Could you check a few things on this model? Use its own coordinates, in mm. A direction names the side the tool comes from. Give positions to 0.01 mm unless a question says otherwise; leave off trailing zeros. Write each loop counter-clockwise with the first axis right and the second up, starting at its lowest first coordinate (ties: lowest second). Pieces come first, ordered by that corner, then holes. Notation, with made-up numbers: (43.5, -12.5) - (73.5, -12.5) arc R11 cw to (73.5, -7.5) - close; hole circle Ø8 at (79.25, 80). An arc over 180 degrees is marked (long way). Use one line per item in the form item = value.
```python
from build123d import *

# Parameters (mm, degrees)
SKETCH1_W           = 76
SKETCH1_H           = 50
BOSS_EXTRUDE1_DEPTH = 20
SKETCH2_W           = 47
SKETCH2_H           = 17
CUT_EXTRUDE1_DEPTH  = 76
SKETCH3_R           = 6.5
CUT_EXTRUDE2_DEPTH  = 2
SKETCH4_R           = 5
CUT_EXTRUDE3_DEPTH  = 2
SKETCH5_R           = 1.2
CUT_EXTRUDE4_DEPTH  = 2


with BuildPart() as part:
    # Sketch1 → Boss-Extrude1 (new body)
    with BuildSketch(Plane(origin=(0, 0, 0), x_dir=(1, 0, 0), z_dir=(0, 1, 0))):
        with Locations((11.529653553, 8.750876438)):
            Rectangle(SKETCH1_W, SKETCH1_H)
    extrude(amount=BOSS_EXTRUDE1_DEPTH)

    # Sketch2 → Cut-Extrude1 (cut)
    with BuildSketch(Plane.ZY.offset(26.470346447)):
        with Locations((-8.750876438, 10)):
            Rectangle(SKETCH2_W, SKETCH2_H)
    extrude(amount=-CUT_EXTRUDE1_DEPTH, mode=Mode.SUBTRACT)

    # Sketch3 → Cut-Extrude2 (cut)
    with BuildSketch(Plane(origin=(0, 0, -33.750876438), x_dir=(-1, 0, 0), z_dir=(0, 0, -1))):
        with Locations((10.970346447, 10)):
            Circle(SKETCH3_R)
        with Locations((-4.029653553, 10)):
            Circle(SKETCH3_R)
        with Locations((-19.029653553, 10)):
            Circle(SKETCH3_R)
        with Locations((-34.029653553, 10)):
            Circle(SKETCH3_R)
    extrude(amount=-CUT_EXTRUDE2_DEPTH, mode=Mode.SUBTRACT)

    # Sketch4 → Cut-Extrude3 (cut)
    with BuildSketch(Plane.XY.offset(16.249123562)):
        with Locations((-10.970346447, 10)):
            Circle(SKETCH4_R)
        with Locations((4.029653553, 10)):
            Circle(SKETCH4_R)
        with Locations((19.029653553, 10)):
            Circle(SKETCH4_R)
        with Locations((34.029653553, 10)):
            Circle(SKETCH4_R)
    extrude(amount=-CUT_EXTRUDE3_DEPTH, mode=Mode.SUBTRACT)

    # Sketch5 → Cut-Extrude4 (cut)
    with BuildSketch(Plane(origin=(0, 0, 0), x_dir=(-1, 0, 0), z_dir=(0, -1, 0))):
        with Locations(Location((-34.029653553, 20.750876438, 0), (0, 0, 90))):  # turned: the seam where the file's is
            Circle(SKETCH5_R)
        with Locations(Location((-19.029653553, 20.750876438, 0), (0, 0, 90))):  # turned: the seam where the file's is
            Circle(SKETCH5_R)
        with Locations(Location((-4.029653553, 20.750876438, 0), (0, 0, 90))):  # turned: the seam where the file's is
            Circle(SKETCH5_R)
        with Locations(Location((10.970346447, 20.750876438, 0), (0, 0, 90))):  # turned: the seam where the file's is
            Circle(SKETCH5_R)
        with Locations(Location((-19.029653553, 5.750876438, 0), (0, 0, 90))):  # turned: the seam where the file's is
            Circle(SKETCH5_R)
        with Locations(Location((-4.029653553, 5.750876438, 0), (0, 0, 90))):  # turned: the seam where the file's is
            Circle(SKETCH5_R)
        with Locations(Location((10.970346447, 5.750876438, 0), (0, 0, 90))):  # turned: the seam where the file's is
            Circle(SKETCH5_R)
        with Locations(Location((-34.029653553, 5.750876438, 0), (0, 0, 90))):  # turned: the seam where the file's is
            Circle(SKETCH5_R)
    extrude(amount=-CUT_EXTRUDE4_DEPTH, mode=Mode.SUBTRACT)


solid = part.part
```
1. If I drill on line 1 (Y direction, x = 21.5, z = 7); line 2 (Z direction, x = 30.5, y = 17.25); line 3 (Z direction, x = -1, y = 9.75), over which ranges is the centre line in solid material (lowest first)? Write a range as from..to.
Response values:
line_1 = 0..1.5, 18.5..20
line_2 = -33.75..-32.25, 14.75..16.25
line_3 = 14.75..16.25
2. If we mould it in two halves opening along Y, with no side actions, what happens to faces 1 (the face through (19.841, 0.74, -19.866)), 2 (the face through (11, 20, -9)), 3 (the face through (38.648, 8.085, 15.51))? For each: pulls with the +Y half, pulls with the -Y half, needs draft (parallel to the pull), parting line crosses it, or undercut.
Response values:
face_1 = needs draft
face_2 = pulls with the +Y half
face_3 = undercut
3. Which directions (+Z, -Z, +X, -X, +Y, -Y) give clear straight access to the entire face, cutting with the end or side of a thin tool? Please do faces 4 (the face through (-12.035, 0.74, -6.305)), 5 (the face through (40.523, 10.286, -33.011)), 6 (the face through (49.53, 19, -7)).
Response values:
face_4 = -Y
face_5 = -Z
face_6 = +Z, -Z, +X, +Y, -Y
4. Imagine slicing it at A-A, the plane z = 9.5. List the corners of the cut face in (x, y) for me.
Response values:
outline = (-26.47, 0) - (49.53, 0) - (49.53, 1.5) - (-26.47, 1.5) - close; (-26.47, 18.5) - (49.53, 18.5) - (49.53, 20) - (-26.47, 20) - close
5. For pin 1 (10.5 mm diameter, centred on x = -10.97, y = 10, fed in from -Z), with a flat end and sliding along its axis, tell me the tip position at first contact or that it passes through.
Response values:
pin_1 = 14.75
6. Imagine slicing it at B-B, the plane y = 10. State how many separate pieces and enclosed holes the cut face has, and give its area (3 significant figures).
Response values:
separate_pieces = 10
enclosed_holes = 0
area = 90.0 mm²
